Source: CAD feature listing. Evaluate the final solid. Frame: model axes, mm. Face numbers are marked on the shaded views. A direction names the side the tool comes from. Round coordinates to 2 decimals unless told otherwise and drop trailing zeros. Loops run counter-clockwise (first coordinate to the right, second up) from the corner with the lowest first, then second, coordinate; pieces in that order, holes last. Notation, with made-up numbers: (89.25, 80) - (108.25, 80) arc R26 ccw to (108.25, 103) - close; hole circle Ø8 at (46, -17.5). An arc over 180 degrees is marked (long way). One line per question, with ' | ' between items. Start each with the question number.
1. Cut plane D-D (x = 7.5). Return loops of the section in (y, z).
2. Mould query, pull axis Y, two halves, no side actions, for the marked faces 4, 5 and 6. Classes: pulls with the +Y half, pulls with the -Y half, needs draft (parallel to the pull), parting line crosses it, or undercut.
3. Ray query, line 1 (Y direction, x = 0, z = 7); line 2 (Z direction, x = -18.5, y = 10); line 3 (Y direction, x = -3, z = 7). Return the intervals inside material, ascending.
4. Pin query (flat end, axial travel): pin 1 (9.5 mm diameter, centred on x = -19, z = 9, fed in from +Y); pin 2 (1.5 mm diameter, centred on x = -11.5, y = -20.5, fed in from +Z); pin 3 (4.5 mm diameter, centred on x = 0, z = 11.5, fed in from -Y). Return the tip coordinate at first contact, or that it passes through.
5. Access query for the marked faces 1, 2 and 3. Directions: +Z, -Z, +X, -X, +Y, -Y. A direction counts if a zero-diameter tool reaches every point of the face in a straight line with its end or side. Return the directions, or none.
6. Cut plane B-B (x = 0). Return loops of the section in (y, z), then the cut area to 3 significant figures.
7. Cut plane A-A (y = 4.5). Return loops of the section in (x, z).
```python
from build123d import *

# Parameters (mm, degrees)
SKETCH_R      = 27.5
SKETCH_R_2    = 22.5
SKETCH_R_3    = 1
PAD_DEPTH     = 10
SKETCH001_R   = 22.5
SKETCH001_R_2 = 14
PAD001_DEPTH  = 4
PAD002_DEPTH  = 2
PAD003_DEPTH  = 2
SKETCH004_R   = 14
SKETCH004_R_2 = 13.5
PAD004_DEPTH  = 16


with BuildPart() as part:
    # Sketch → Pad (new body)
    with BuildSketch(Plane.XY):
        Circle(SKETCH_R)
        Circle(SKETCH_R_2, mode=Mode.SUBTRACT)
        with Locations((0, 25)):
            Circle(SKETCH_R_3, mode=Mode.SUBTRACT)
        with Locations((-21.650635, -12.5)):
            Circle(SKETCH_R_3, mode=Mode.SUBTRACT)
        with Locations((21.650635, -12.5)):
            Circle(SKETCH_R_3, mode=Mode.SUBTRACT)
    extrude(amount=PAD_DEPTH)

    # Sketch001 → Pad001 (join)
    with BuildSketch(Plane.XY):
        Circle(SKETCH001_R)
        Circle(SKETCH001_R_2, mode=Mode.SUBTRACT)
    extrude(amount=PAD001_DEPTH)

    # Sketch002 → Pad002 (join, symmetric)
    with BuildSketch(Plane.XZ):
        Polygon((22.5, 10), (22.5, 4), (13, 4), (13, 16), align=None)
        Polygon((-22.5, 10), (-22.5, 4), (-13, 4), (-13, 16), align=None)
    extrude(amount=PAD002_DEPTH, both=True)

    # Sketch003 → Pad003 (join, symmetric)
    with BuildSketch(Plane.YZ):
        Polygon((13, 4), (22.5, 4), (22.5, 10), (13, 16), align=None)
        Polygon((-13, 4), (-22.5, 4), (-22.5, 10), (-13, 16), align=None)
    extrude(amount=PAD003_DEPTH, both=True)

    # Sketch004 → Pad004 (join)
    with BuildSketch(Plane.XY):
        Circle(SKETCH004_R)
        Circle(SKETCH004_R_2, mode=Mode.SUBTRACT)
    extrude(amount=PAD004_DEPTH)


solid = part.part
```
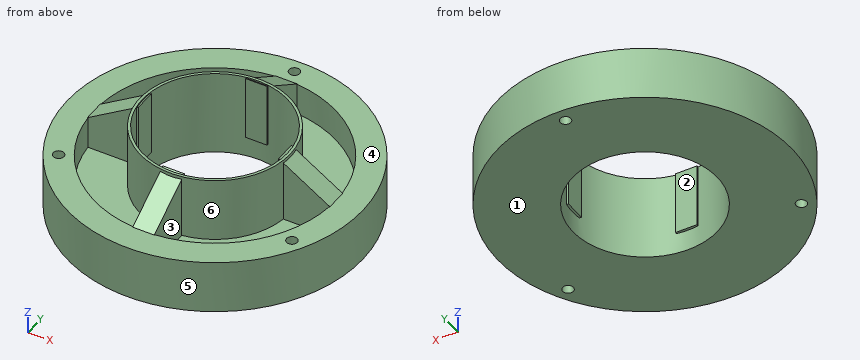
Answers follow:
1) outline: (-26.46, 0) - (-11.22, 0) - (-11.22, 16) - (-11.82, 16) - (-11.82, 4) - (-21.21, 4) - (-21.21, 10) - (-26.46, 10) - close; (11.22, 0) - (26.46, 0) - (26.46, 10) - (21.21, 10) - (21.21, 4) - (11.82, 4) - (11.82, 16) - (11.22, 16) - close
2) face 4: needs draft | face 5: parting line crosses it | face 6: undercut
3) line 1: y = -27.5 to -13, 13 to 24, 26 to 27.5 | line 2: z = 0 to 4 | line 3: y = -27.34 to -22.3, -13.67 to -13.16, 13.16 to 13.67, 22.3 to 27.34
4) pin 1: stops at y = 23.52 | pin 2: stops at z = 10 | pin 3: stops at y = -27.5
5) face 1: -Z, +X, -X, +Y, -Y | face 2: +Z, -Z | face 3: +Z
6) outline: (-27.5, 0) - (-13.5, 0) - (-13.5, 4) - (-13, 4) - (-13, 16) - (-13.5, 15.68) - (-13.5, 16) - (-14, 16) - (-14, 15.37) - (-22.5, 10) - (-27.5, 10) - close; (13, 4) - (13.5, 4) - (13.5, 0) - (24, 0) - (24, 10) - (22.5, 10) - (14, 15.37) - (14, 16) - (13.5, 16) - (13.5, 15.68) - (13, 16) - close; (26, 0) - (27.5, 0) - (27.5, 10) - (26, 10) - close | area: 323 mm2
7) outline: (-27.13, 0) - (-12.73, 0) - (-12.73, 16) - (-13.26, 16) - (-13.26, 4) - (-22.05, 4) - (-22.05, 10) - (-27.13, 10) - close; (12.73, 0) - (27.13, 0) - (27.13, 10) - (22.05, 10) - (22.05, 4) - (13.26, 4) - (13.26, 16) - (12.73, 16) - close
